Autodesk Inventor part; units mm, degrees
ref_plane "YZ Plane" through (0, 0, 0) normal (1, 0, 0) x (0, 1, 0)
ref_plane "XZ Plane" through (0, 0, 0) normal (0, 1, 0) x (-1, 0, 0)
ref_plane "XY Plane" through (0, 0, 0) normal (0, 0, 1) x (1, 0, 0)
sketch "スケッチ1" plane through (0, 0, 0) normal (0, 0, 1) x (1, 0, 0)
  line L0 (2.8284, 0) -> (0, -2.8284)
  line L1 (0, -2.8284) -> (-2.8284, 0)
  line L2 (-2.8284, 0) -> (0, 2.8284)
  line L3 (0, 2.8284) -> (2.8284, 0)
  line L4 (-12.1149, 7.5) -> (-10, -7.5)
  line L5 (10, -7.5) -> (-10, -7.5)
  line L6 (10, -7.5) -> (12.1149, 7.5)
  line L7 (12.1149, 7.5) -> (-12.1149, 7.5)
  point P0 (0, 0)
  point P1 (0, 7.5)
  point P2 (11.0574, 0)
  dimension "d10" = 24.2298
  dimension "d11" = 20
  dimension "d12" = 15
  dimension "d13" = 4
extrude "押し出し1" add sketch "スケッチ1" against normal blind 2
sketch "スケッチ3" plane through (0, 0, 0) normal (0, 0, 1) x (1, 0, 0)
  line L0 (2.8284, 0) -> (0, -2.8284)
  line L1 (0, -2.8284) -> (-2.8284, 0)
  line L2 (-2.8284, 0) -> (0, 2.8284)
  line L3 (0, 2.8284) -> (2.8284, 0)
  circle A0 centre (0, 0) radius 4
  dimension "d17" = 8
extrude "押し出し3" add sketch "スケッチ3" along normal blind 5
sketch "スケッチ4" plane through (0, 0, 5) normal (0, 0, 1) x (1, 0, 0)
  circle A0 centre (0, 0) radius 4
  circle A1 centre (0, 0) radius 4
  line L0 (-1.2, 3.8158) -> (-1.2, 12.5)
  line L1 (-1.2, 12.5) -> (1.2, 12.5)
  line L2 (1.2, 12.5) -> (1.2, 3.8158)
  line L3 (12.1149, 7.5) -> (-12.1149, 7.5) construction
  dimension "d18" = 5
  dimension "d19" = 2.4
extrude "押し出し4" add sketch "スケッチ4" against normal up to surface (7 mm away) contours A0 L0 L1 L2
sketch "スケッチ5" plane through (1.2, 3.8158, 5) normal (1, 0, 0) x (0, 0, -1)
  line L0 (7, 3.6842) -> (7, 8.6842)
  line L1 (0, 8.6842) -> (7, 8.6842)
  line L2 (0, 0) -> (0, 8.6842)
  arc A0 (7, 5.1842) -> (0, 5.1842) centre (3.5, 5.1842) ccw
  point P0 (5, -3.8158)
  point P1 (3.5, 8.6842)
extrude "押し出し5" cut sketch "スケッチ5" along normal through all both and the other way through all
sketch "スケッチ7" plane through (0, 0, 0) normal (0, 0, 1) x (1, 0, 0)
  line L0 (-1.2, 3.8158) -> (-1.2, 7.5)
  line L1 (-1.2, 7.5) -> (-12.1149, 7.5)
  line L2 (-12.1149, 7.5) -> (-10, -7.5)
  line L3 (-10, -7.5) -> (10, -7.5)
  line L4 (10, -7.5) -> (12.1149, 7.5)
  line L5 (12.1149, 7.5) -> (1.2, 7.5)
  line L6 (1.2, 7.5) -> (1.2, 3.8158)
  arc A0 (-1.2, 3.8158) -> (1.2, 3.8158) centre (0, 0) ccw
properties part number "om_BackHolder_V3"
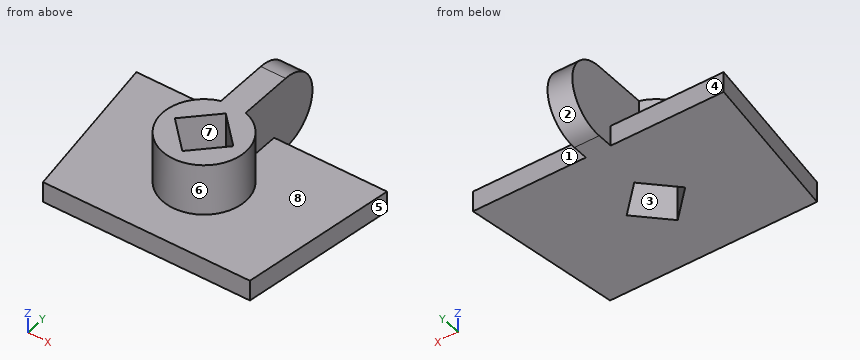
Part model, mm, in its own coordinate system. Face numbers are marked on the shaded views. A direction names the side the tool comes from. Give positions to 0.01 mm unless a question says otherwise; leave off trailing zeros. Loops run counter-clockwise (first coordinate to the right, second up) from the corner with the lowest first, then second, coordinate; pieces in that order, holes last. Notation, with made-up numbers: M -5.75,-1.75 L 2.25,-1.75 A11 ccw 2.25,10.25 Z; hole C -36,62.25 d4. An arc over 180 degrees is marked long. Put each result on its own line as item: value. Start each with the question number.
1) 3-axis set-ups, long thin cutter, end or side, ignore diameter. For the marked faces 1, 2, 3 and 4: which of +Z, -Z, +X, -X, +Y, -Y reach the whole face in a straight line?
2) Saw through at B-B (z = 1). List the corners of the cut face in (x, y), then the cut area to 3 significant figures.
3) Probe probe 1 along Z at (x, y) = (4.5, -5.75); probe 2 along X at (y, z) = (8, 3.5); probe 3 along Y at (x, z) = (8.25, -1). List the from-to ranges inside material, lowest first.
4) Pull direction X, two halves, no side cores. Call the marked faces 5, 6, 7 and 8: +X half, -X half, draft (parallel to the pull), parting line (faces both ways), or undercut.
5) Saw through at C-C (y = 1.25). List the corners of the cut face in (x, z), then the cut area to 3 significant figures.
6) Flat gauge pins, fed straight in: pin 1 (4 mm diameter, centred on x = -6.5, z = 2.5, fed in from -Y); pin 2 (1.5 mm diameter, centred on x = -3.5, z = 3.5, fed in from -Y); pin 3 (1 mm diameter, centred on x = -0.5, z = 3.5, fed in from +Y); pin 4 (2 mm diameter, centred on x = 6, z = -1, fed in from +Y). Where does each tip first touch, or does it go through?
7) Saw through at D-D (y = 3.25). List the corners of the cut face in (x, z), then the cut area to 3 significant figures.
8) Saw through at A-A (x = -1.5). List the corners of the cut face in (y, z).
Numbers:
1. face 1: +Z, -Z, +X, +Y
1. face 2: +X, -X, +Y
1. face 3: +Z, -Z
1. face 4: +Z, -Z, -X, +Y
2. outline: M -1.2,3.82 A4 ccw long 1.2,3.82 L 1.2,12.46 L -1.2,12.46 Z; hole M -2.83,0 L 0,-2.83 L 2.83,0 L 0,2.83 Z
2. area: 54.7 mm^2
3. probe 1: -2 to 0
3. probe 2: -1.2 to 1.2
3. probe 3: -7.5 to 7.5
4. face 5: +X half
4. face 6: parting line
4. face 7: undercut
4. face 8: draft
5. outline: M -11.23,-2 L -1.58,-2 L -1.58,5 L -3.8,5 L -3.8,0 L -11.23,0 Z; M 1.58,-2 L 11.23,-2 L 11.23,0 L 3.8,0 L 3.8,5 L 1.58,5 Z
5. area: 60.8 mm^2
6. pin 1: through
6. pin 2: y = -2.9
6. pin 3: y = 12.16
6. pin 4: y = 7.5
7. outline: M -11.52,-2 L 11.52,-2 L 11.52,0 L 2.33,0 L 2.33,5 L -2.33,5 L -2.33,0 L -11.52,0 Z
7. area: 69.4 mm^2
8. outline: M -7.5,-2 L -1.33,-2 L -1.33,5 L -3.71,5 L -3.71,0 L -7.5,0 Z; M 1.33,-2 L 7.5,-2 L 7.5,0 L 3.71,0 L 3.71,5 L 1.33,5 Z
